The model under review builds one solid part; all positions refer to its coordinate system, in mm. A direction names the side the tool comes from. Coordinates: 2 decimals unless noted, no trailing zeros. Write each loop counter-clockwise with the first axis right and the second up, starting at its lowest first coordinate (ties: lowest second). Pieces come first, ordered by that corner, then holes. Notation, with made-up numbers: (22, 14.25) -> (69, 14.25) arc R26 ccw to (69, 34.25) -> close; hole circle Ø7 at (-23.75, 43.25). An arc over 180 degrees is marked (long way). Write each question's results on one line, items separated by ' | '.
```python
from build123d import *

# Parameters (mm, degrees)
EXTRUDE_1_DEPTH              = 6
SKETCH_2_R                   = 28.5
CUT_EXTRUDE_1_DEPTH          = 1
HOLE_START                   = 2.6
HOLE_WIZARD_M3_1_OUTLINE_R   = 3
HOLE_WIZARD_M3_1_DEPTH       = 3.4
HOLE_START_2                 = 1
HOLE_WIZARD_M3_1_2_OUTLINE_R = 1.7
HOLE_WIZARD_M3_1_2_DEPTH     = 1.6


# Read off the part's stored shape, not the designer's step: M3 六角圆柱头螺钉的柱形沉头孔1
with BuildPart() as part:
    # 草图1 → 凸台-拉伸1 (new body)
    with BuildSketch(Plane.XY):
        with BuildLine():
            Line((0, 30), (30, 30))
            Line((30, 30), (30, -30))
            Line((30, -30), (0, -30))
            ThreePointArc((0, -30), (-30, 0), (0, 30))
        make_face()
    extrude(amount=EXTRUDE_1_DEPTH)

    # 草图2 → 切除-拉伸1 (cut)
    with BuildSketch(Plane(origin=(0, 0, 0), x_dir=(-1, 0, 0), z_dir=(0, 0, -1))):
        Circle(SKETCH_2_R)
    extrude(amount=-CUT_EXTRUDE_1_DEPTH, mode=Mode.SUBTRACT)

    # M3 六角圆柱头螺钉的柱形沉头孔1 outline → M3 六角圆柱头螺钉的柱形沉头孔1 (cut)
    with BuildSketch(Plane.XY.offset(HOLE_START)):
        with Locations((13.435028843, 13.435028843)):
            Circle(HOLE_WIZARD_M3_1_OUTLINE_R)
        with Locations((-13.435028843, -13.435028843)):
            Circle(HOLE_WIZARD_M3_1_OUTLINE_R)
        with Locations((-13.435028843, 13.435028843)):
            Circle(HOLE_WIZARD_M3_1_OUTLINE_R)
        with Locations((13.435028843, -13.435028843)):
            Circle(HOLE_WIZARD_M3_1_OUTLINE_R)
        Circle(HOLE_WIZARD_M3_1_OUTLINE_R)
    extrude(amount=HOLE_WIZARD_M3_1_DEPTH, mode=Mode.SUBTRACT)

    # Hole Wizard M3 _1 2 outline → Hole Wizard M3 _1 2 (cut)
    with BuildSketch(Plane.XY.offset(HOLE_START_2)):
        with Locations((13.435028843, 13.435028843)):
            Circle(HOLE_WIZARD_M3_1_2_OUTLINE_R)
        with Locations((-13.435028843, -13.435028843)):
            Circle(HOLE_WIZARD_M3_1_2_OUTLINE_R)
        with Locations((-13.435028843, 13.435028843)):
            Circle(HOLE_WIZARD_M3_1_2_OUTLINE_R)
        with Locations((13.435028843, -13.435028843)):
            Circle(HOLE_WIZARD_M3_1_2_OUTLINE_R)
        Circle(HOLE_WIZARD_M3_1_2_OUTLINE_R)
    extrude(amount=HOLE_WIZARD_M3_1_2_DEPTH, mode=Mode.SUBTRACT)


solid = part.part
```
Q1. Clearance check with flat-ended pins moving along their axes: P1, Ø3.5, axis at x = 13.44, y = 13.44, coming from the -Z side; P2, Ø5.5, axis at x = 13.44, y = 13.44, coming from the +Z side; P3, Ø2.5, axis at x = -13.44, y = -13.44, coming from the +Z side. State where each tip first meets the part, or that it passes through.
Solution:
P1: z = 1 | P2: z = 2.6 | P3: through
Q2. Draft analysis for pull direction X (two halves, no side actions). For faces 1 (the flat face through (30, 0, 3)), 2 (the cylindrical face through (-26.327, -10.916, 0.493)), 3 (the flat face through (15, -30, 3)), state which applies: pulls with the +X half, pulls with the -X half, needs draft (parallel to the pull), parting line crosses it, or undercut.
Solution:
face 1: pulls with the +X half | face 2: undercut | face 3: needs draft
Q3. Machinability: for faces 4 (the cylindrical face through (-0.37, -1.66, 1.79)), 5 (the flat face through (0, -6, 1)), 6 (the flat face through (15, 12, 2.6)), which of the approach directions +Z, -Z, +X, -X, +Y, -Y give a long, thin tool a straight path to every point of the face, cutting with its end or side? Answer none if there is none.
Solution:
face 4: +Z, -Z | face 5: -Z | face 6: +Z
Q4. For line 1 (Z direction, x = -9, y = 19); line 2 (Y direction, x = -2, z = 0.95); line 3 (X direction, y = -1, z = 4.4), list the stretches that pass through material, from the lowest coordinate up. Write a range as from..to.
Solution:
line 1: 1..6 | line 2: -29.93..-28.43, 28.43..29.93 | line 3: -29.98..-2.83, 2.83..30
Q5. Add section C-C (x = 19). Write out the cut boundary in (y, z).
Solution:
outline: (-30, 0) -> (-21.24, 0) -> (-21.24, 1) -> (21.24, 1) -> (21.24, 0) -> (30, 0) -> (30, 6) -> (-30, 6) -> close
Q6. Add section D-D (y = -20). Write out the cut boundary in (x, z).
Solution:
outline: (-22.36, 0) -> (-20.3, 0) -> (-20.3, 1) -> (20.3, 1) -> (20.3, 0) -> (30, 0) -> (30, 6) -> (-22.36, 6) -> close
Q7. Add section A-A (y = 0). Write out the cut boundary in (x, z), plus the area to 3 significant figures.
Solution:
outline: (-30, 0) -> (-28.5, 0) -> (-28.5, 1) -> (-1.7, 1) -> (-1.7, 2.6) -> (-3, 2.6) -> (-3, 6) -> (-30, 6) -> close; (1.7, 1) -> (28.5, 1) -> (28.5, 0) -> (30, 0) -> (30, 6) -> (3, 6) -> (3, 2.6) -> (1.7, 2.6) -> close | area: 277 mm²
Q8. Add section B-B (z = 1.7). Write out the cut boundary in (x, y), plus the area to 3 significant figures.
Solution:
outline: (0, -30) -> (30, -30) -> (30, 30) -> (0, 30) arc R30 ccw to start; hole circle Ø3.4 at (-13.44, -13.44); hole circle Ø3.4 at (-13.44, 13.44); hole circle Ø3.4 at (0, 0); hole circle Ø3.4 at (13.44, -13.44); hole circle Ø3.4 at (13.44, 13.44) | area: 3,170 mm²
